Could you check a few things on this model? Use its own coordinates, in mm. Face numbers are marked on the shaded views. A direction names the side the tool comes from. Coordinates: 2 decimals unless noted, no trailing zeros. Write each loop counter-clockwise with the first axis right and the second up, starting at its lowest first coordinate (ties: lowest second). Pieces come first, ordered by that corner, then holes. Notation, with made-up numbers: (36.25, 31) - (58.25, 31) arc R29 ccw to (58.25, 57) - close; hole circle Ø7 at (20, 11.5). An arc over 180 degrees is marked (long way). Answer as a JSON object with one key per item and string values. Group by question number.
1) If we section it at C-C (y = 0): Write out the boundary of the cut face in (x, z).
2) We'd pull the mould along X, two halves only. Please class the marked faces 1, 2 and 3: released by +X, released by -X, zero draft, split by the parting line, or undercut.
3) Will these pins go through, and if not, where does the flat tip stop? pin 1 Ø15 at (x, y) = (-2, -7) entering from +Z; pin 2 Ø12 at (x, y) = (0, 0) entering from -Z.
4) If we section it at B-B (z = 20): Write out the boundary of the cut face in (x, y).
5) If we section it at A-A (x = 0): Write out the boundary of the cut face in (y, z).
6) Please list where these lines run through material, in increasing order: line 1 along X through (y, z) = (-12, 20); line 2 along Y through (x, z) = (0, 14.25).
7) On a 3-axis mill with a long thin cutter (end or side, diameter ignored), from which of +Z, -Z, +X, -X, +Y, -Y can I reach the whole of each face in a straight line? I mean the marked faces 4 and 5. Say none if no direction works.
```python
from build123d import *

# Parameters (mm, degrees)
F0_W     = 30
F0_H     = 30
F1_DEPTH = 49.1
F2_R     = 6.75
F3_DEPTH = 22
F4_W     = 2
F4_H     = 2
F5_DEPTH = 1
F8_R     = 1.5
F9_DEPTH = 8.4197768095


with BuildPart() as f1:
    # F0 (on Top) → F1 (new body)
    with BuildSketch(Plane.XY):
        Rectangle(F0_W, F0_H)
    extrude(amount=F1_DEPTH)

    # F2 (on Top) → F3 (cut)
    with BuildSketch(Plane.XY):
        Circle(F2_R)
    extrude(amount=F3_DEPTH, mode=Mode.SUBTRACT)

    # F4 (on face) → F5 (join)
    with BuildSketch(Plane.XY.offset(49.1)):
        with Locations((14, 14)):
            Rectangle(F4_W, F4_H)
        with Locations((14, -14)):
            Rectangle(F4_W, F4_H)
        with Locations((-14, -14)):
            Rectangle(F4_W, F4_H)
        with Locations((-14, 14)):
            Rectangle(F4_W, F4_H)
    extrude(amount=F5_DEPTH)

    # F6 (on Front) → F7 (revolve, cut)
    with BuildSketch(Plane.XZ):
        Polygon((0, 14.9834286422), (0, 0), (10, 0), align=None)
    revolve(axis=Axis((0, 0, 7.4917143211), (0, 0, -1)), mode=Mode.SUBTRACT)

    # F8 (on face) → F9 (cut, through all)
    with BuildSketch(Plane.XZ.offset(15)):
        with Locations((0, 20)):
            Circle(F8_R)
    extrude(amount=-F9_DEPTH, mode=Mode.SUBTRACT)


solid = f1.part
```
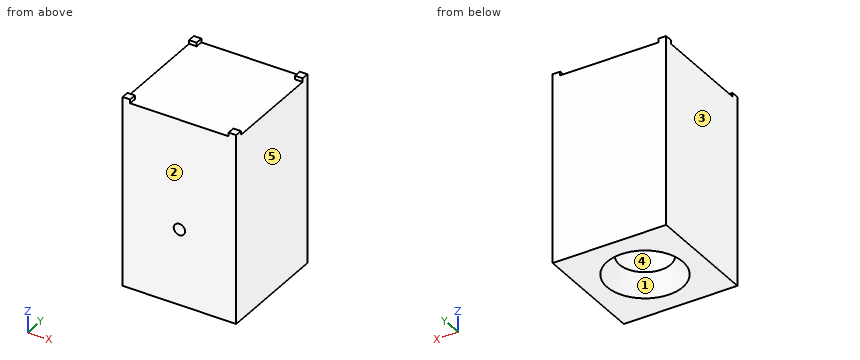
Here are the results:
{
 "1": {"outline": "(-15, 0) - (-10, 0) - (-6.75, 4.87) - (-6.75, 22) - (6.75, 22) - (6.75, 4.87) - (10, 0) - (15, 0) - (15, 49.1) - (-15, 49.1) - close"},
 "2": {"face 1": "undercut", "face 2": "zero draft", "face 3": "released by -X"},
 "3": {"pin 1": "stops at z = 49.1", "pin 2": "stops at z = 22"},
 "4": {"outline": "(-15, -15) - (-1.5, -15) - (-1.5, -6.58) arc R6.75 cw (long way) to (1.5, -6.58) - (1.5, -15) - (15, -15) - (15, 15) - (-15, 15) - close"},
 "5": {"outline": "(-15, 0) - (-10, 0) - (-6.75, 4.87) - (-6.75, 18.5) - (-15, 18.5) - close; (-15, 21.5) - (-6.75, 21.5) - (-6.75, 22) - (6.75, 22) - (6.75, 4.87) - (10, 0) - (15, 0) - (15, 49.1) - (-15, 49.1) - close"},
 "6": {"line 1": "x = -15 to -1.5, 1.5 to 15", "line 2": "y = -15 to -6.75, 6.75 to 15"},
 "7": {"face 4": "-Z", "face 5": "+Z, -Z, +X, +Y, -Y"}
}
